Model file for the job. Use its own axes, mm. Face numbers are marked on the shaded views. A direction names the side the tool comes from. Round coordinates to 2 decimals unless told otherwise and drop trailing zeros. Loops run counter-clockwise (first coordinate to the right, second up) from the corner with the lowest first, then second, coordinate; pieces in that order, holes last. Notation, with made-up numbers: (57.25, 81.25) -> (71.25, 81.25) arc R29 cw to (71.25, 112.25) -> close; hole circle Ø9 at (-22.5, 74). An arc over 180 degrees is marked (long way). Use a Markdown table: item, result. Add a question column.
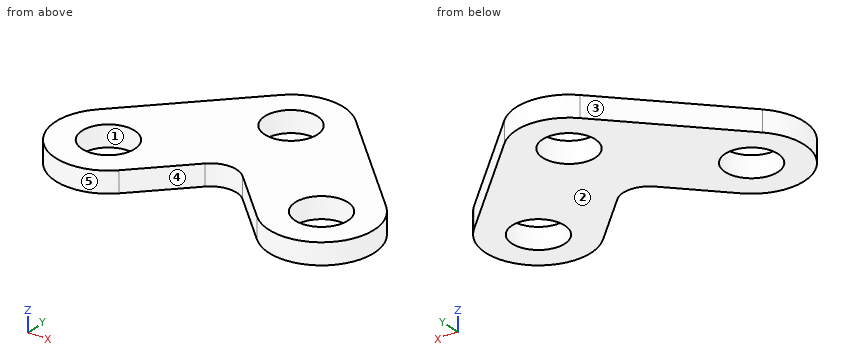
```python
from build123d import *

# Parameters (mm, degrees)
SM_BASE_FLANGE_1_DEPTH = 4
SKETCH_6_R             = 5
CUT_EXTRUDE_1_DEPTH    = 10
FILLET_1_R             = 5


# Sheet-metal steps are written as plain solids
with BuildPart() as part:
    # Sketch 1 → 基体-法兰1 (new body)
    with BuildSketch(Plane.XY):
        with BuildLine():
            Line((-7.071067812, 7.071067812), (-27.071067812, -12.928932188))
            ThreePointArc((-27.071067812, -12.928932188), (-27.071067812, -27.071067812), (-12.928932188, -27.071067812))
            Line((-12.928932188, -27.071067812), (0, -14.142135624))
            Line((0, -14.142135624), (12.928932188, -27.071067812))
            ThreePointArc((12.928932188, -27.071067812), (27.071067812, -27.071067812), (27.071067812, -12.928932188))
            Line((27.071067812, -12.928932188), (7.071067812, 7.071067812))
            ThreePointArc((7.071067812, 7.071067812), (0, 10), (-7.071067812, 7.071067812))
        make_face()
    extrude(amount=-SM_BASE_FLANGE_1_DEPTH)

    # 草图6 → 切除-拉伸1 (cut)
    with BuildSketch(Plane.XY):
        Circle(SKETCH_6_R)
        with Locations((-20, -20)):
            Circle(SKETCH_6_R)
        with Locations((20, -20)):
            Circle(SKETCH_6_R)
    extrude(amount=-CUT_EXTRUDE_1_DEPTH, mode=Mode.SUBTRACT)

    # 圆角1
    fillet_1_edges = [part.edges().sort_by_distance(p)[0] for p in [
        (0, -14.142135624, -2),
    ]]
    fillet(fillet_1_edges, radius=FILLET_1_R)


solid = part.part
```
1) Tool access for the marked faces 4 and 5: list every direction of +Z, -Z, +X, -X, +Y, -Y with a clear straight run to the whole face (end or side of a thin tool).
2) Cut at C-C on y = 1.5. Write the cut outline in (x, z).
3) Pin check, flat tips, straight feed: pin 1 Ø1.5 at (y, z) = (-3.5, -2) entering from -X; pin 2 Ø1.5 at (y, z) = (-3, -2.5) entering from -X. Stop position of each tip, or through.
4) Cut at B-B on x = 0. Write the cut outline in (y, z), and give its area (3 significant figures).
5) Wall check: probe 1 along X at (y, z) = (-23, -2.95); probe 2 along X at (y, z) = (-22.5, -1.15); probe 3 along Y at (x, z) = (0, -2.1). Give the ranges that are in metal, low to high. Write a range as from..to.
6) Cut at D-D on y = -20. Write the cut outline in (x, z).
7) Pull direction X, two halves, no side cores. Call the marked faces 1, 2 and 3: +X half, -X half, draft (parallel to the pull), parting line (faces both ways), or undercut.
Established:
| question | item | result |
|---|---|---|
| 1 | face 4 | +Z, -Z, -Y |
| 1 | face 5 | +Z, -Z |
| 2 | outline | (-12.64, -4) -> (-4.77, -4) -> (-4.77, 0) -> (-12.64, 0) -> close; (4.77, -4) -> (12.64, -4) -> (12.64, 0) -> (4.77, 0) -> close |
| 3 | pin 1 | stops at x = -18.39 |
| 3 | pin 2 | stops at x = -17.89 |
| 4 | outline | (-16.21, -4) -> (-5, -4) -> (-5, 0) -> (-16.21, 0) -> close; (5, -4) -> (10, -4) -> (10, 0) -> (5, 0) -> close |
| 4 | area | 64.9 mm^2 |
| 5 | probe 1 | x = -29.54..-24, -16..-8.86, 8.86..16, 24..29.54 |
| 5 | probe 2 | x = -29.68..-24.33, -15.67..-8.36, 8.36..15.67, 24.33..29.68 |
| 5 | probe 3 | y = -16.21..-5, 5..10 |
| 6 | outline | (-30, -4) -> (-25, -4) -> (-25, 0) -> (-30, 0) -> close; (-15, -4) -> (-5.86, -4) -> (-5.86, 0) -> (-15, 0) -> close; (5.86, -4) -> (15, -4) -> (15, 0) -> (5.86, 0) -> close; (25, -4) -> (30, -4) -> (30, 0) -> (25, 0) -> close |
| 7 | face 1 | undercut |
| 7 | face 2 | draft |
| 7 | face 3 | -X half |
